from build123d import *

# Parameters (mm, degrees)
SKETCH_1_R      = 9
SKETCH_1_R_2    = 6
EXTRUDE_1_DEPTH = 4
CHAMFER_1_SIZE  = 0.1
EXTRUDE_START   = -0.8
SKETCH_2_R      = 9.75
SKETCH_2_R_2    = 6
EXTRUDE_2_DEPTH = 0.8


with BuildPart() as part:
    # 草图1 → 凸台-拉伸1 (new body)
    with BuildSketch(Plane.XY):
        Circle(SKETCH_1_R)
        Circle(SKETCH_1_R_2, mode=Mode.SUBTRACT)
    extrude(amount=EXTRUDE_1_DEPTH)

    # 倒角1
    chamfer_1_edges = [part.edges().sort_by_distance(p)[0] for p in [
        (-9, 0, 0),
        (-6, 0, 0),
    ]]
    chamfer(chamfer_1_edges, length=CHAMFER_1_SIZE)

    # 草图2 → 凸台-拉伸2 (add)
    with BuildSketch(Plane.XY.offset(4).offset(EXTRUDE_START)):
        Circle(SKETCH_2_R)
        Circle(SKETCH_2_R_2, mode=Mode.SUBTRACT)
    extrude(amount=EXTRUDE_2_DEPTH)


solid = part.part
Source: CAD feature listing. Evaluate the final solid. Frame: model axes, mm. A direction names the side the tool comes from. Round coordinates to 2 decimals unless told otherwise and drop trailing zeros. Order: outer loops, then holes, each group sorted by start corner. A loop starts at its lowest first (then second) coordinate and runs counter-clockwise, first axis right, second up. Notation, with made-up numbers: (3.5, 32.5) -> (33.5, 32.5) arc R13 ccw to (33.5, 52.5) -> close; hole circle Ø11 at (61.5, 29.25). An arc over 180 degrees is marked (long way). Answer as CSV lines item,"result".
Item 1: Section C-C, the plane z = 1.8. Return loops of the section in (x, y).
A:
outline,"circle Ø18 at (0, 0); hole circle Ø12 at (0, 0)"
Item 2: Reachability of faces 4 (the face through (-4.5, -4.2, 4)), 5 (the face through (3, -9, 3.2)) from +Z, -Z, +X, -X, +Y, -Y: full face, straight path, thin tool, end or side. Return the list, or none.
A:
face 4,"+Z, +X, -X, +Y, -Y"
face 5,"-Z"
Item 3: Pin query (flat end, axial travel): pin 1 Ø1 at (y, z) = (-6, 1.5) entering from -X; pin 2 Ø11 at (x, y) = (0, 0) entering from +Z. Return the tip coordinate at first contact, or that it passes through.
A:
pin 1,"x = -7.12"
pin 2,"through"
Item 4: Pull-direction query (X, two-part tool) for faces 1 (the face through (6, 2, 0)), 2 (the face through (-1.172, 8.923, 1.628)), 3 (the face through (-6, 0, 2)); classes: pulls with the +X half, pulls with the -X half, needs draft (parallel to the pull), parting line crosses it, or undercut.
A:
face 1,"needs draft"
face 2,"parting line crosses it"
face 3,"undercut"
Item 5: Line query: L1, parallel to Y at x = 0, z = 1.1; L2, parallel to Y at x = -5.5, z = 1.6; L3, parallel to X at y = -6.5, z = 0.2. Output: solid intervals per line, ascending.
A:
L1,"-9 to -6, 6 to 9"
L2,"-7.12 to -2.4, 2.4 to 7.12"
L3,"-6.22 to 6.22"
Item 6: Section A-A, the plane x = 0. Return loops of the section in (y, z), plus the area to 3 significant figures.
A:
outline,"(-9.75, 3.2) -> (-9, 3.2) -> (-9, 0.1) -> (-8.9, 0) -> (-6.1, 0) -> (-6, 0.1) -> (-6, 4) -> (-9.75, 4) -> close; (6, 0.1) -> (6.1, 0) -> (8.9, 0) -> (9, 0.1) -> (9, 3.2) -> (9.75, 3.2) -> (9.75, 4) -> (6, 4) -> close"
area,"25.2 mm²"
